from build123d import *

# Parameters (mm, degrees)
BOSS_EXTRUDE1_DEPTH = 1.6
SKETCH2_W           = 80.5
SKETCH2_H           = 16
BOSS_EXTRUDE2_DEPTH = 13
CUT_EXTRUDE1_REACH  = 69.621
SKETCH3_R           = 2
CHAMFER1_SIZE       = 1.5
SKETCH4_W           = 6
SKETCH4_H           = 11
BOSS_EXTRUDE3_DEPTH = 12
SKETCH5_W           = 4
SKETCH5_H           = 2
BOSS_EXTRUDE4_DEPTH = 6


with BuildPart() as part:
    # Sketch1 → Boss-Extrude1 (new body)
    with BuildSketch(Plane(origin=(0, 0, 0), x_dir=(1, 0, 0), z_dir=(0, 1, 0))):
        Polygon((-44.75, 45.5), (44.75, 45.5), (44.75, -45.5), (34.75, -45.5), (33.75, -46.5), (-33.75, -46.5), (-34.75, -45.5), (-44.75, -45.5), align=None)
    extrude(amount=BOSS_EXTRUDE1_DEPTH)

    # Sketch2 → Boss-Extrude2 (add)
    with BuildSketch(Plane(origin=(0, 1.6, 0), x_dir=(1, 0, 0), z_dir=(0, 1, 0))):
        with Locations((-3.5, 41)):
            Rectangle(SKETCH2_W, SKETCH2_H)
    extrude(amount=BOSS_EXTRUDE2_DEPTH)

    # Sketch3 → Cut-Extrude1 (cut, up to next)
    with BuildSketch(Plane(origin=(0, 1.6, 0), x_dir=(1, 0, 0), z_dir=(0, 1, 0)), mode=Mode.PRIVATE) as cut_extrude1_sk1:
        with Locations(Location((-35.25, -37, 0), (0, 0, 270))):
            Circle(SKETCH3_R)
    cut_extrude1_tool1 = extrude(cut_extrude1_sk1.sketch, amount=-CUT_EXTRUDE1_REACH, mode=Mode.PRIVATE) & part.part
    # Sketch3 → Cut-Extrude1 (cut, up to next)
    with BuildSketch(Plane(origin=(0, 1.6, 0), x_dir=(1, 0, 0), z_dir=(0, 1, 0)), mode=Mode.PRIVATE) as cut_extrude1_sk2:
        with Locations(Location((35.25, -37, 0), (0, 0, 270))):
            Circle(SKETCH3_R)
    cut_extrude1_tool2 = extrude(cut_extrude1_sk2.sketch, amount=-CUT_EXTRUDE1_REACH, mode=Mode.PRIVATE) & part.part
    add(cut_extrude1_tool1.solids().sort_by_distance((-35.25, 1.6, 37))[0], mode=Mode.SUBTRACT)
    add(cut_extrude1_tool2.solids().sort_by_distance((35.25, 1.6, 37))[0], mode=Mode.SUBTRACT)

    # Chamfer1
    chamfer1_edges = [part.edges().sort_by_distance(p)[0] for p in [
        (44.75, 0.8, 45.5),
        (-44.75, 0.8, 45.5),
    ]]
    chamfer(chamfer1_edges, length=CHAMFER1_SIZE)

    # Sketch4 → Boss-Extrude3 (add)
    with BuildSketch(Plane(origin=(0, 1.6, 0), x_dir=(1, 0, 0), z_dir=(0, 1, 0))):
        with Locations((41.35, 37.5)):
            Rectangle(SKETCH4_W, SKETCH4_H)
    extrude(amount=BOSS_EXTRUDE3_DEPTH)

    # Sketch5 → Boss-Extrude4 (add)
    with BuildSketch(Plane(origin=(0, 0, -43), x_dir=(-1, 0, 0), z_dir=(0, 0, -1))):
        with Locations((-41.35, 4.8)):
            Rectangle(SKETCH5_W, SKETCH5_H)
    extrude(amount=BOSS_EXTRUDE4_DEPTH)


solid = part.part
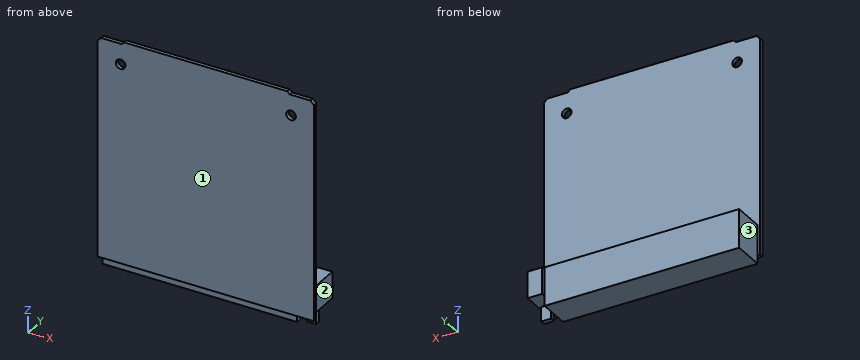
Check sheet for the modelled part. Datum: model origin and axes. Units: mm. Face numbers are marked on the shaded views. A direction names the side the tool comes from. Give positions to 0.01 mm unless a question says otherwise; leave off trailing zeros. Write each loop counter-clockwise with the first axis right and the second up, starting at its lowest first coordinate (ties: lowest second). Pieces come first, ordered by that corner, then holes. Notation, with made-up numbers: (49, -22) -> (56, -22) arc R17 ccw to (56, 7) -> close; hole circle Ø3 at (75.5, 0.5). An arc over 180 degrees is marked (long way). Use one line per item in the form item = value. Start each with the question number.
1. Thickness scan on line 1 along X through (y, z) = (1.15, 37); line 2 along Z through (x, y) = (-20, 11.25); line 3 along Y through (x, z) = (34, -12.5). Record the ranges inside material, lowest first. Write a range as from..to.
2. Go/stop test with flat-tipped pins: P1, Ø3, axis at x = 42, y = 10.5, coming from the -Z side; P2, Ø6.5, axis at x = 41.5, z = -40, coming from the +Y side; P3, Ø6, axis at x = 8.5, y = 6.5, coming from the +Z side. Record where each tip stops, or that it passes through.
3. Access from +Z, -Z, +X, -X, +Y, -Y to the whole of each face (thin tool, end or side, straight path). Record for the marked faces 1, 2 and 3.
4. Section check B-B (x = 9.5). Record the cut outline in (y, z).
5. Section check A-A (z = 37). Record the cut outline in (x, y).
Conclusion:
q1.line_1 = -44.75..-37.25, -33.25..33.25, 37.25..44.75
q1.line_2 = -49..-33
q1.line_3 = 0..1.6
q2.P1 = -43
q2.P2 = 13.6
q2.P3 = -33
q3.face_1 = +Z, -Z, +X, -X, -Y
q3.face_2 = +Z, -Z, +X, +Y
q3.face_3 = +Z, -Z, -X, +Y
q4.outline = (0, -45.5) -> (1.6, -45.5) -> (1.6, -49) -> (14.6, -49) -> (14.6, -33) -> (1.6, -33) -> (1.6, 46.5) -> (0, 46.5) -> close
q5.outline = (-44.75, 0) -> (-37.25, 0) -> (-37.25, 1.6) -> (-44.75, 1.6) -> close; (-33.25, 0) -> (33.25, 0) -> (33.25, 1.6) -> (-33.25, 1.6) -> close; (37.25, 0) -> (44.75, 0) -> (44.75, 1.6) -> (37.25, 1.6) -> close
